Verification items for the finished model (mm, model axes). Face numbers are marked on the shaded views. A direction names the side the tool comes from. Round coordinates to 2 decimals unless told otherwise and drop trailing zeros. Write each loop counter-clockwise with the first axis right and the second up, starting at its lowest first coordinate (ties: lowest second). Pieces come first, ordered by that corner, then holes. Notation, with made-up numbers: M -38,-26.75 L -26,-26.75 A10 ccw -26,-14.75 Z; hole C 69.25,-25.75 d9. An arc over 180 degrees is marked long. Answer in a Markdown table with one row per item. Add a question column.
1. Sectioned sample at A-A on z = 0. Record the cut outline in (x, y), plus the area to 3 significant figures.
2. Sectioned sample at B-B on y = 36. Record the cut outline in (x, z).
3. Material ranges on probe 1 along Z at (x, y) = (-8, 36); probe 2 along Y at (x, z) = (1, -55); probe 3 along Y at (x, z) = (7, 0), recorded low to high.
4. Go/stop test with flat-tipped pins: pin 1 Ø4 at (y, z) = (18.5, 12.5) entering from +X; pin 2 Ø18 at (y, z) = (12.5, -87.5) entering from +X; pin 3 Ø12 at (x, z) = (11, -25) entering from -Y. Record where each tip stops, or that it passes through.
5. Draft check along Y on the marked faces 1, 2 and 3. Enter one of: pulls with the +Y half, pulls with the -Y half, needs draft (parallel to the pull), parting line crosses it, or undercut.
6. Sectioned sample at C-C on x = 0. Record the cut outline in (y, z).
7. Sectioned sample at D-D on z = -111. Record the cut outline in (x, y).
8. Set-up check for the marked faces 4, 5 and 6: record each of +Z, -Z, +X, -X, +Y, -Y from which the full face is reachable in a straight line by a thin tool's end or side.
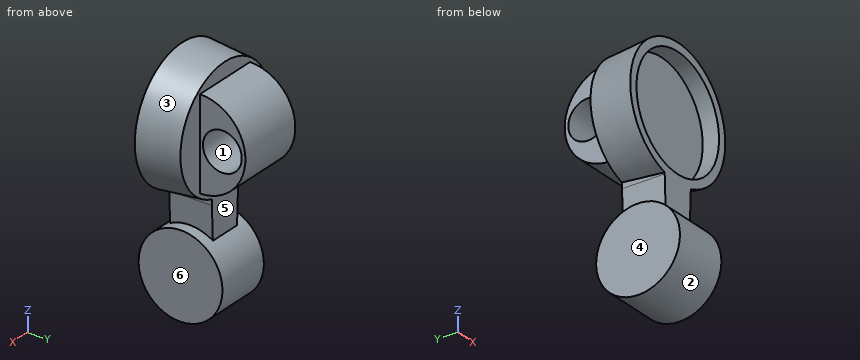
```python
from build123d import *

# Parameters (mm, degrees)
BOSS_EXTRUDE1_DEPTH      = 24.380571
BOSS_EXTRUDE1_DEPTH_BACK = 24.380571
SKETCH2_R                = 13.935202
BOSS_EXTRUDE2_DEPTH      = 30.655768
BOSS_EXTRUDE3_DEPTH      = 20.236561
BOSS_EXTRUDE3_DEPTH_BACK = 20.236561
SKETCH5_R                = 30.106112


with BuildPart() as part:
    # Sketch1 → Revolve1 (revolve)
    with BuildSketch(Plane.XY, mode=Mode.PRIVATE) as revolve1_sk:
        Polygon((-40.3145498, 0), (-46.3804, 0), (-43.5102, 30.655768), (0, 30.655768), (0, 11.70178), (-40.3145498, 11.70178), align=None)
    revolve(revolve1_sk.sketch.rotate(Axis((0, 0, 0), (0, -1, 0)), 270), axis=Axis((0, 0, 0), (0, -1, 0)))

    # Sketch2 → Boss-Extrude1 (add, two sides: drawn at the far end of the back side and taken through both)
    with BuildSketch(Plane(origin=(0, 0, 0), x_dir=(0, 0, -1), z_dir=(1, 0, 0)).offset(-BOSS_EXTRUDE1_DEPTH_BACK)):
        with BuildLine():
            Line((0, 30.655768), (-32.625284, 30.655768))
            ThreePointArc((-32.625284, 30.655768), (0, 63.281052), (32.625284, 30.655768))
            Line((32.625284, 30.655768), (0, 30.655768))
        make_face()
        with Locations((0, 46.734476)):
            Circle(SKETCH2_R, mode=Mode.SUBTRACT)
    extrude(amount=BOSS_EXTRUDE1_DEPTH + BOSS_EXTRUDE1_DEPTH_BACK)

    # Sketch4 → Boss-Extrude2 (add)
    with BuildSketch(Plane(origin=(0, 0, 0), x_dir=(1, 0, 0), z_dir=(0, 1, 0))):
        Polygon((12.72794, 45.609256), (10.780776, 95.954596), (-10.780776, 95.954596), (-12.72794, 45.609256), (-12.927645356, 40.445728926), (12.927645356, 40.445728926), align=None)
    extrude(amount=BOSS_EXTRUDE2_DEPTH)

    # Sketch5 → Boss-Extrude3 (add, two sides: drawn at the far end of the back side and taken through both)
    with BuildSketch(Plane(origin=(0, 0, 0), x_dir=(0, 0, -1), z_dir=(1, 0, 0)).offset(-BOSS_EXTRUDE3_DEPTH_BACK)):
        with Locations((94.013528, 13.638022)):
            Circle(SKETCH5_R)
    extrude(amount=BOSS_EXTRUDE3_DEPTH + BOSS_EXTRUDE3_DEPTH_BACK)


solid = part.part
```
Geometry check:
| question | item | result |
|---|---|---|
| 1 | outline | M -46.38,0 L -40.31,0 L -40.31,11.7 L 40.31,11.7 L 40.31,0 L 46.38,0 L 43.51,30.66 L 24.38,30.66 L 24.38,32.8 L -24.38,32.8 L -24.38,30.66 L -43.51,30.66 Z; M -24.38,60.67 L 24.38,60.67 L 24.38,63.28 L -24.38,63.28 Z |
| 1 | area | 2,040 mm2 |
| 2 | outline | M -24.38,-32.18 L 24.38,-32.18 L 24.38,-8.89 L -24.38,-8.89 Z; M -24.38,8.89 L 24.38,8.89 L 24.38,32.18 L -24.38,32.18 Z; M -20.24,-114.17 L 20.24,-114.17 L 20.24,-73.86 L -20.24,-73.86 Z |
| 3 | probe 1 | z = -114.17 to -73.86, -32.18 to -8.89, 8.89 to 32.18 |
| 3 | probe 2 | y = 0 to 30.66 |
| 3 | probe 3 | y = 11.7 to 32.8, 60.67 to 63.28 |
| 4 | pin 1 | stops at x = 43.43 |
| 4 | pin 2 | stops at x = 20.24 |
| 4 | pin 3 | stops at y = 11.7 |
| 5 | face 1 | undercut |
| 5 | face 2 | parting line crosses it |
| 5 | face 3 | pulls with the +Y half |
| 6 | outline | M 0,-67.17 A30.11 ccw long 30.66,-69.18 L 30.66,-32.63 A32.63 ccw 30.66,32.63 L 30.66,43.51 L 0,46.38 L 0,40.31 L 11.7,40.31 L 11.7,-40.31 L 0,-40.31 Z; hole C 46.73,0 d27.87 |
| 7 | outline | M -20.24,-11.22 L 20.24,-11.22 L 20.24,38.49 L -20.24,38.49 Z |
| 8 | face 4 | -Z, -X, +Y, -Y |
| 8 | face 5 | +Y |
| 8 | face 6 | -Z, +X, +Y, -Y |
